Source: CAD feature listing. Evaluate the final solid. Frame: model axes, mm. A direction names the side the tool comes from. Round coordinates to 2 decimals unless told otherwise and drop trailing zeros. Loops run counter-clockwise (first coordinate to the right, second up) from the corner with the lowest first, then second, coordinate; pieces in that order, holes last. Notation, with made-up numbers: (67, 73.5) - (113, 73.5) arc R11 cw to (113, 78.5) - close; hole circle Ø10 at (64.25, 88). An arc over 180 degrees is marked (long way). One line per question, with ' | ' between items.
from build123d import *

# Parameters (mm, degrees)
MAIN_BODY_DEPTH            = 16
SKETCH8_W                  = 134
SKETCH8_H                  = 4
COVER_DEPTH                = 72
SKETCH20_W                 = 116
SKETCH20_H                 = 14
CRYSTAL_SLOT_DEPTH         = 65
SKETCH9_W                  = 14
SKETCH9_H                  = 14
SIPM_WINDOW_DEPTH          = 14
TUBE_ADAPTER_DEPTH         = 30
RIGHT_SCREW_TERMINAL_DEPTH = 10
RIGHT_SCREW_HOLE_REACH     = 136
SKETCH12_R                 = 1.524
LEFT_SCREW_TERMINAL_DEPTH  = 10
LEFT_SCREW_HOLE_REACH      = 136
SKETCH14_R                 = 1.524
ADAPTER_HOLE_REACH         = 146
SKETCH18_R                 = 1.524
SKETCH21_W                 = 54
SKETCH21_H                 = 54
FILTER_SLOT_DEPTH          = 2.7
SKETCH24_W                 = 49
SKETCH24_H                 = 49
FILTER_WINDOW_DEPTH        = 1.8


with BuildPart() as part:
    # Sketch5 → Main Body (new body)
    with BuildSketch(Plane(origin=(0, 0, 0), x_dir=(1, 0, 0), z_dir=(0, 1, 0))):
        Polygon((-134, 0), (-124, 0), (-1.95326153, 0), (0, 0), (0, 72), (-134, 72), align=None)
    extrude(amount=-MAIN_BODY_DEPTH)

    # Sketch8 → Cover (add)
    with BuildSketch(Plane.XY):
        with Locations((-67, -18)):
            Rectangle(SKETCH8_W, SKETCH8_H)
    extrude(amount=-COVER_DEPTH)

    # Sketch20 → Crystal Slot (cut)
    with BuildSketch(Plane.XY):
        with Locations((-62, -11.5)):
            Rectangle(SKETCH20_W, SKETCH20_H)
    extrude(amount=-CRYSTAL_SLOT_DEPTH, mode=Mode.SUBTRACT)

    # Sketch9 → SiPM Window (cut)
    with BuildSketch(Plane.ZY.offset(134)):
        with Locations((-36, -11.5)):
            Rectangle(SKETCH9_W, SKETCH9_H)
    extrude(amount=-SIPM_WINDOW_DEPTH, mode=Mode.SUBTRACT)

    # Sketch10 → Tube Adapter (add)
    with BuildSketch(Plane.XZ.offset(20)):
        with BuildLine():
            Line((-134, -13), (-134, -16))
            ThreePointArc((-134, -16), (-114, -36), (-134, -56))
            Line((-134, -56), (-134, -59))
            ThreePointArc((-134, -59), (-111, -36), (-134, -13))
        make_face()
    extrude(amount=TUBE_ADAPTER_DEPTH)

    # Sketch11 → Right Screw Terminal (add)
    with BuildSketch(Plane.XZ.offset(20)):
        with BuildLine():
            Line((-134, -59), (-134, -69))
            Line((-134, -69), (-124, -69))
            Line((-124, -69), (-124, -56.712315177))
            ThreePointArc((-124, -56.712315177), (-128.870830919, -58.420785547), (-134, -59))
        make_face()
    extrude(amount=RIGHT_SCREW_TERMINAL_DEPTH)

    # Sketch12 → Right Screw Hole (cut, up to next)
    with BuildSketch(Plane.ZY.offset(134), mode=Mode.PRIVATE) as right_screw_hole_sk1:
        with Locations((-64, -25)):
            Circle(SKETCH12_R)
    right_screw_hole_tool1 = extrude(right_screw_hole_sk1.sketch, amount=-RIGHT_SCREW_HOLE_REACH, mode=Mode.PRIVATE) & part.part
    add(right_screw_hole_tool1.solids().sort_by_distance((-134, -25, -64))[0], mode=Mode.SUBTRACT)

    # Sketch13 → Left Screw Terminal (add)
    with BuildSketch(Plane(origin=(0, -20, 0), x_dir=(-1, 0, 0), z_dir=(0, -1, 0))):
        with BuildLine():
            Line((134, 13), (134, 3))
            Line((134, 3), (124, 3))
            Line((124, 3), (124, 15.287684823))
            ThreePointArc((124, 15.287684823), (128.870830919, 13.579214453), (134, 13))
        make_face()
    extrude(amount=LEFT_SCREW_TERMINAL_DEPTH)

    # Sketch14 → Left Screw Hole (cut, up to next)
    with BuildSketch(Plane.ZY.offset(134), mode=Mode.PRIVATE) as left_screw_hole_sk1:
        with Locations((-8, -25)):
            Circle(SKETCH14_R)
    left_screw_hole_tool1 = extrude(left_screw_hole_sk1.sketch, amount=-LEFT_SCREW_HOLE_REACH, mode=Mode.PRIVATE) & part.part
    add(left_screw_hole_tool1.solids().sort_by_distance((-134, -25, -8))[0], mode=Mode.SUBTRACT)

    # Sketch18 → Adapter Hole (cut, up to next)
    with BuildSketch(Plane.ZY.offset(144), mode=Mode.PRIVATE) as adapter_hole_sk1:
        with Locations((-36, -42.5)):
            Circle(SKETCH18_R)
    adapter_hole_tool1 = extrude(adapter_hole_sk1.sketch, amount=-ADAPTER_HOLE_REACH, mode=Mode.PRIVATE) & part.part
    add(adapter_hole_tool1.solids().sort_by_distance((-144, -42.5, -36))[0], mode=Mode.SUBTRACT)

    # Sketch21 → Filter Slot (cut)
    with BuildSketch(Plane.XZ.offset(4.5)):
        with Locations((-33.5, -36)):
            Rectangle(SKETCH21_W, SKETCH21_H)
        with Locations((-90, -36)):
            Rectangle(SKETCH21_W, SKETCH21_H)
    extrude(amount=-FILTER_SLOT_DEPTH, mode=Mode.SUBTRACT)

    # Sketch24 → Filter Window (cut)
    with BuildSketch(Plane.XZ.offset(1.8)):
        with Locations((-33.5, -36)):
            Rectangle(SKETCH24_W, SKETCH24_H)
        with Locations((-90, -36)):
            Rectangle(SKETCH24_W, SKETCH24_H)
    extrude(amount=-FILTER_WINDOW_DEPTH, mode=Mode.SUBTRACT)


solid = part.part
1. Contact query for flat-ended pins moving along their axis: P1, Ø5, axis at x = -48.5, z = -48.5, coming from the -Y side; P2, Ø6, axis at y = -31.5, z = -51.5, coming from the -X side; P3, Ø1.5, axis at y = -36.5, z = -22, coming from the -X side. Output: stop coordinate, or through.
Worked out:
P1: stops at y = -20 | P2: stops at x = -126.4 | P3: stops at x = -120.49
2. Section query A-A, the plane y = -14.5. Return loops of the section in (x, z), plus the area to 3 significant figures.
Worked out:
outline: (-134, -72) - (0, -72) - (0, 0) - (-4, 0) - (-4, -65) - (-120, -65) - (-120, -43) - (-134, -43) - close; (-134, -29) - (-120, -29) - (-120, 0) - (-134, 0) - close | area: 1,910 mm2
3. Section query D-D, the plane z = -36. Give the number of separate pieces and of enclosed holes in the cut face, plus the area to 3 significant figures.
Worked out:
separate pieces: 4 | enclosed holes: 0 | area: 473 mm2
4. Access query for faces 1 (the flat face through (-34, -3, -9)), 2 (the flat face through (-4, -12, -32)), 3 (the cylindrical face through (-111.006, -34.79, -36.506)), 4 (the flat face through (-124, -25, -62)). Directions: +Z, -Z, +X, -X, +Y, -Y. A direction counts if a zero-diameter tool reaches every point of the face in a straight line with its end or side. Return the directions, or none.
Worked out:
face 1: none | face 2: +Z | face 3: +X, -Y | face 4: -Z, +X, -Y
5. Material intervals for probe 1 along Y at (x, z) = (-118, -47); probe 2 along Y at (x, z) = (-128, -64); probe 3 along X at (y, z) = (-17, -28), sorted ascending.
Worked out:
probe 1: y = -20 to -18.5, -4.5 to 0 | probe 2: y = -30 to -26.52, -23.48 to 0 | probe 3: x = -134 to -120, -4 to 0
6. Section query B-B, the plane x = -42.5. Return loops of the section in (y, z), plus the area to 3 significant figures.
Worked out:
outline: (-20, -72) - (0, -72) - (0, -60.5) - (-1.8, -60.5) - (-1.8, -63) - (-4.5, -63) - (-4.5, -65) - (-18.5, -65) - (-18.5, 0) - (-20, 0) - close; (-4.5, -9) - (-1.8, -9) - (-1.8, -11.5) - (0, -11.5) - (0, 0) - (-4.5, 0) - close | area: 296 mm2
7. Mould query, pull axis X, two halves, no side actions, for faces 5 (the flat face through (-70, -18.5, -33)), 6 (the flat face through (-124, -25, -10)), 7 (the cylindrical face through (-114, -35, -36)). Classes: released by +X, released by -X, zero draft, split by the parting line, or undercut.
Worked out:
face 5: undercut | face 6: released by +X | face 7: released by -X
8. Section query C-C, the plane z = -23. Return loops of the section in (x, y), plus the area to 3 significant figures.
Worked out:
outline: (-134, -20) - (-118.8, -20) - (-118.8, -50) - (-115.03, -50) - (-115.03, -20) - (0, -20) - (0, 0) - (-9, 0) - (-9, -1.8) - (-6.5, -1.8) - (-6.5, -4.5) - (-4, -4.5) - (-4, -18.5) - (-120, -18.5) - (-120, -4.5) - (-117, -4.5) - (-117, -1.8) - (-114.5, -1.8) - (-114.5, 0) - (-134, 0) - close; (-65.5, -1.8) - (-63, -1.8) - (-63, -4.5) - (-60.5, -4.5) - (-60.5, -1.8) - (-58, -1.8) - (-58, 0) - (-65.5, 0) - close | area: 701 mm2
